Could you check a few things on this drawing? It's one solid part, dimensions in mm from its lowest x, y, z. A direction names the side the tool comes from. Give positions to 0.01 mm unless a question says otherwise; leave off trailing zeros. Loops run counter-clockwise (first coordinate to the right, second up) from the corner with the lowest first, then second, coordinate; pieces in that order, holes last.
Q1. I need wall thicknesses on probe 1 along Y at (x, z) = (205, 40); probe 2 along Y at (x, z) = (231, 123); probe 3 along Z at (x, y) = (38, 109). Which ranges of each line are inside material? Lowest first, please.
Q2. For the marked faces 1, 2 and 3, which set-ups out of +Z, -Z, +X, -X, +Y, -Y let a thin tool reach every point of the face, with its end or its side?
Q3. Suppose I cut it at C-C (x = 205). List the corners of the cut face in (y, z) for me.
Q4. Suppose I cut it at B-B (z = 125). List the corners of the cut face in (x, y) for me, and give its area (3 significant figures).
Q5. Suppose I cut it at D-D (x = 110.5). List the corners of the cut face in (y, z) for me.
Q6. Suppose I cut it at A-A (y = 85). List the corners of the cut face in (x, z) for me, and give its area (3 significant figures).
Q7. I'm going to push flat-ended pins straight in: P1, Ø20, axis at y = 65.5, z = 286, coming from the +X side; P2, Ø1, axis at x = 217, y = 37, coming from the +Z side; P3, Ø1, axis at y = 72, z = 112, coming from the +X side. Where does each tip first touch, or does it pass through?
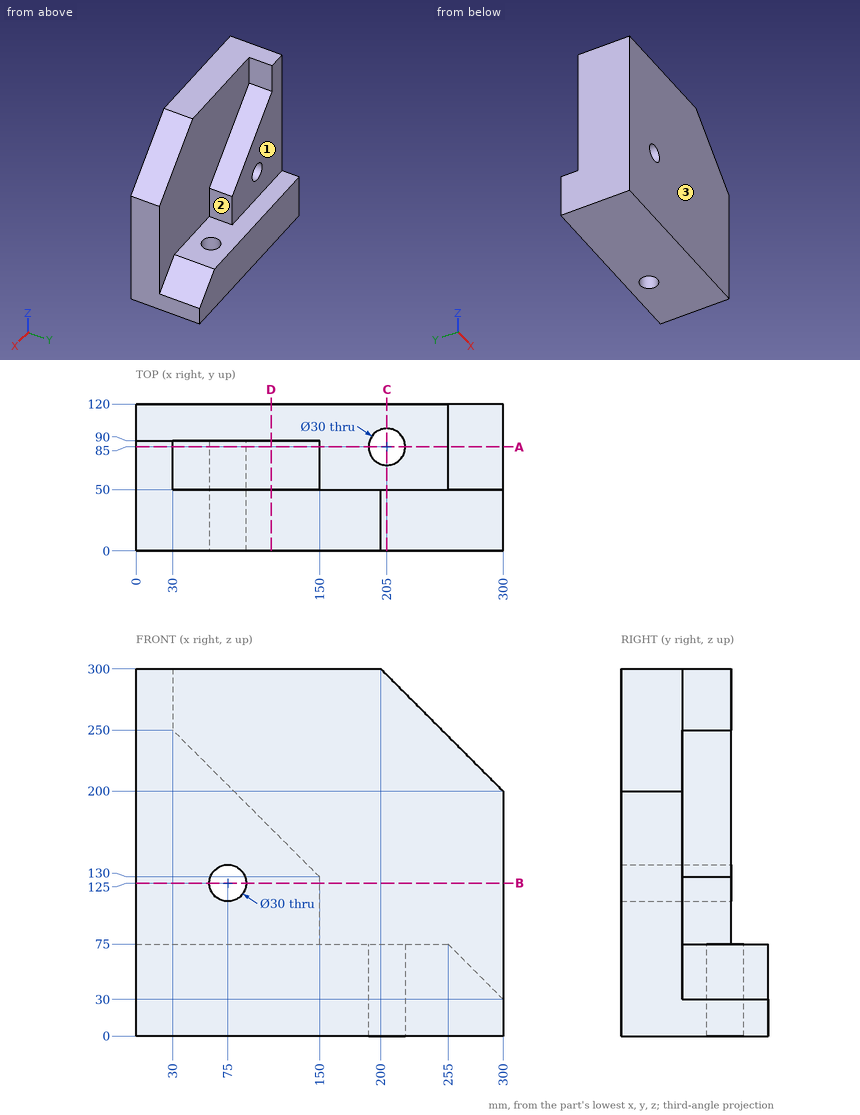
Solutions:
1. probe 1: y = 0 to 70, 100 to 120
1. probe 2: y = 0 to 50
1. probe 3: z = 0 to 75
2. face 1: +Z, +X, -X, +Y
2. face 2: +Z, +X, +Y
2. face 3: +Z, -Z, +X, -X, -Y
3. outline: (0, 0) - (70, 0) - (70, 75) - (50, 75) - (50, 295) - (0, 295) - close; (100, 0) - (120, 0) - (120, 75) - (100, 75) - close
4. outline: (0, 0) - (60, 0) - (60, 90) - (0, 90) - close; (90, 0) - (300, 0) - (300, 50) - (150, 50) - (150, 90) - (90, 90) - close
4. area: 18,300 mm2
5. outline: (0, 0) - (120, 0) - (120, 75) - (90, 75) - (90, 169.5) - (50, 169.5) - (50, 300) - (0, 300) - close
6. outline: (0, 0) - (190, 0) - (190, 75) - (150, 75) - (150, 130) - (30, 250) - (30, 300) - (0, 300) - close; (220, 0) - (300, 0) - (300, 30) - (255, 75) - (220, 75) - close; hole circle Ø30 at (75, 125)
6. area: 39,100 mm2
7. P1: stops at x = 30
7. P2: stops at z = 283.5
7. P3: stops at x = 150
